Read the model definition and answer for the solid it produces. Units are mm, in the model's axes. A direction names the side the tool comes from. Give positions to 0.01 mm unless a question says otherwise; leave off trailing zeros. Order: outer loops, then holes, each group sorted by start corner. A loop starts at its lowest first (then second) coordinate and runs counter-clockwise, first axis right, second up. Notation, with made-up numbers: M -16.75,33 L 21.25,33 A19 cw 21.25,51 Z; hole C 14.5,43.5 d4. An arc over 180 degrees is marked long. One line per item, written item: value. Start each with the question number.
from build123d import *

# Parameters (mm, degrees)
SCHIZZO1_R                   = 1.5
ESTRUSIONE_ESTRUSIONE1_DEPTH = 4
SMUSSO1_SIZE                 = 0.25
RACCORDO4_R                  = 1
RACCORDO5_R                  = 1


with BuildPart() as part:
    # Schizzo1 → Estrusione-Estrusione1 (new body)
    with BuildSketch(Plane.XY):
        with BuildLine():
            Line((0, 0), (22.720595315, 0))
            ThreePointArc((22.720595315, 0), (29.560998181, 1.206147584), (35.576347508, 4.679111138))
            Line((35.576347508, 4.679111138), (65.894780202, 30.119296829))
            ThreePointArc((65.894780202, 30.119296829), (69.422068894, 33.968656964), (71.832880424, 38.599782825))
            Line((71.832880424, 38.599782825), (77.25204587, 53.48881752))
            ThreePointArc((77.25204587, 53.48881752), (76.217545127, 58.601179223), (71.195710383, 60.011005371))
            Line((71.195710383, 60.011005371), (71.083987609, 59.979479494))
            ThreePointArc((71.083987609, 59.979479494), (66.995210403, 57.683229946), (64.402806168, 53.775506658))
            Line((64.402806168, 53.775506658), (60.906270246, 44.168853168))
            ThreePointArc((60.906270246, 44.168853168), (58.495458716, 39.537727307), (54.968170024, 35.688367172))
            Line((54.968170024, 35.688367172), (29.930313668, 14.679111138))
            ThreePointArc((29.930313668, 14.679111138), (23.91496434, 11.206147584), (17.074561474, 10))
            Line((17.074561474, 10), (0, 10))
            Line((0, 10), (0, 0))
        make_face()
        with Locations((15, 5)):
            Circle(SCHIZZO1_R, mode=Mode.SUBTRACT)
    extrude(amount=-ESTRUSIONE_ESTRUSIONE1_DEPTH)

    # Smusso1
    smusso1_edges = [part.edges().sort_by_distance(p)[0] for p in [
        (13.5, 5, 0),
        (13.5, 5, -4),
    ]]
    chamfer(smusso1_edges, length=SMUSSO1_SIZE)

    # Raccordo4
    raccordo4_edges = [part.edges().sort_by_distance(p)[0] for p in [
        (74.542463147, 46.044300172, -4),
        (76.217545127, 58.601179223, -4),
        (71.139848996, 59.995242433, -4),
        (66.995210403, 57.683229946, -4),
        (62.654538207, 48.972179913, -4),
        (58.495458716, 39.537727307, -4),
        (42.449241846, 25.183739155, -4),
        (23.91496434, 11.206147584, -4),
        (8.537280737, 10, -4),
        (11.360297657, 0, -4),
        (29.560998181, 1.206147584, -4),
        (50.735563855, 17.399203983, -4),
        (69.422068894, 33.968656964, -4),
    ]]
    fillet(raccordo4_edges, radius=RACCORDO4_R)

    # Raccordo5
    raccordo5_edges = [part.edges().sort_by_distance(p)[0] for p in [
        (69.422068894, 33.968656964, 0),
        (50.735563855, 17.399203983, 0),
        (29.560998181, 1.206147584, 0),
        (11.360297657, 0, 0),
        (8.537280737, 10, 0),
        (23.91496434, 11.206147584, 0),
        (42.449241846, 25.183739155, 0),
        (58.495458716, 39.537727307, 0),
        (62.654538207, 48.972179913, 0),
        (66.995210403, 57.683229946, 0),
        (71.139848996, 59.995242433, 0),
        (76.217545127, 58.601179223, 0),
        (74.542463147, 46.044300172, 0),
    ]]
    fillet(raccordo5_edges, radius=RACCORDO5_R)


solid = part.part
Q1. Find section A-A, the plane x = 15. Give the vertices of the cut face in (y, z).
Q2. Each of these flat-tipped pins is pushed along its axis until it touches: pin 1 (1.5 mm diameter, centred on x = 43.5, z = -2.5, fed in from +Y); pin 2 (2 mm diameter, centred on x = 12.5, z = -1.5, fed in from +Y). Where does it stop, or does it pass through?
Q3. Consider probe 1 along Y at (x, z) = (15, -1.45); probe 2 along Y at (x, z) = (68, -2.55); probe 3 along Y at (x, z) = (67, -0.4). Determine where each line is inside the solid, lowest interval first.
Q4. Find section B-B, the plane z = -1.75. Give the vertices of the cut face in (x, y), then the cut area to 3 significant figures.
Q5. A tool of negligible diameter and unlimited length cuts with its end or side. For faces 4 (the cylindrical face through (62.913, 48.802, -3.715)), 5 (the flat face through (9, 10, -2)), from which of +Z, -Z, +X, -X, +Y, -Y can it reach the whole face along a straight path? Write none if from no direction.
Q6. Determine the mould class of faces 1 (the cylindrical face through (13.5, 5.07, -1.98)), 2 (the flat face through (44, 24, -4)), 3 (the cylindrical face through (29.469, 1.173, -1.986)) for opening direction X: released by +X, released by -X, zero draft, split by the parting line, or undercut.
Evaluation:
1. outline: M 0,-3 A1 ccw 1,-4 L 3.25,-4 L 3.5,-3.75 L 3.5,-0.25 L 3.25,0 L 1,0 A1 ccw 0,-1 Z; M 6.5,-3.75 L 6.75,-4 L 9,-4 A1 ccw 10,-3 L 10,-1 A1 ccw 9,0 L 6.75,0 L 6.5,-0.25 Z
2. pin 1: y = 26.69
2. pin 2: y = 10
3. probe 1: 0 to 3.5, 6.5 to 10
3. probe 2: 32.17 to 58.5
3. probe 3: 31.4 to 57.41
4. outline: M 0,0 L 22.72,0 A20 ccw 35.58,4.68 L 65.89,30.12 A20 ccw 71.83,38.6 L 77.25,53.49 A5 ccw 71.2,60.01 L 71.08,59.98 A10 ccw 64.4,53.78 L 60.91,44.17 A20 cw 54.97,35.69 L 29.93,14.68 A20 cw 17.07,10 L 0,10 Z; hole C 15,5 d3
4. area: 1,100 mm2
5. face 4: -Z, -X, +Y
5. face 5: +Z, -Z, -X, +Y
6. face 1: undercut
6. face 2: zero draft
6. face 3: released by +X
